The model under review builds one solid part; all positions refer to its coordinate system, in mm. Face numbers are marked on the shaded views. Give positions to 0.01 mm unless a question says otherwise; leave off trailing zeros. Write each loop counter-clockwise with the first axis right and the second up, starting at its lowest first coordinate (ties: lowest second). Pieces come first, ordered by that corner, then holes. Notation, with made-up numbers: (9, 79.25) -> (16, 79.25) arc R23 cw to (16, 106.25) -> close; hole circle Ø10 at (-0.75, 6). An arc over 180 degrees is marked (long way). Use CSV: the item, a comma, the result in double quotes.
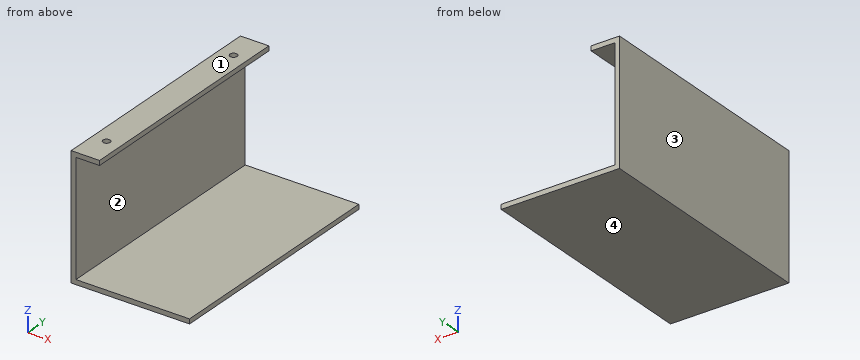
```python
from build123d import *

# Parameters (mm, degrees)
F0_W     = 50
F0_H     = 100
F1_DEPTH = 2
F2_W     = 2
F2_H     = 100
F3_DEPTH = 50
F4_W     = 100
F4_H     = 2
F5_DEPTH = 10
F6_R     = 1.5
F7_DEPTH = 2


with BuildPart() as f1:
    # F0 (on Top) → F1 (new body)
    with BuildSketch(Plane.XY):
        Rectangle(F0_W, F0_H)
    extrude(amount=F1_DEPTH)

    # F2 (on face) → F3 (join)
    with BuildSketch(Plane.XY.offset(2)):
        with Locations((-24, 0)):
            Rectangle(F2_W, F2_H)
    extrude(amount=F3_DEPTH)

    # F4 (on face) → F5 (join)
    with BuildSketch(Plane.YZ.offset(-23)):
        with Locations((0, 51)):
            Rectangle(F4_W, F4_H)
    extrude(amount=F5_DEPTH)

    # F6 (on face) → F7 (cut, through all)
    with BuildSketch(Plane.XY.offset(52)):
        with Locations((-18.9944, 37.5)):
            Circle(F6_R)
        with Locations((-18.9944, -37.5)):
            Circle(F6_R)
    extrude(amount=-F7_DEPTH, mode=Mode.SUBTRACT)


solid = f1.part
```
Q1. Consider section B-B (y = 25.5). Write out the cut boundary in (x, z), then the cut area to 3 significant figures.
Derived:
outline,"(-25, 0) -> (25, 0) -> (25, 2) -> (-23, 2) -> (-23, 50) -> (-13, 50) -> (-13, 52) -> (-25, 52) -> close"
area,"220 mm2"
Q2. The part is to be moulded in two halves that separate along Z. For the marked faces 1, 2, 3 and 4, say which applies: pulls with the +Z half, pulls with the -Z half, needs draft (parallel to the pull), parting line crosses it, or undercut.
Derived:
face 1,"pulls with the +Z half"
face 2,"undercut"
face 3,"needs draft"
face 4,"pulls with the -Z half"
Q3. Consider section C-C (x = -19). Write out the cut boundary in (y, z).
Derived:
outline,"(-50, 0) -> (50, 0) -> (50, 2) -> (-50, 2) -> close; (-50, 50) -> (-39, 50) -> (-39, 52) -> (-50, 52) -> close; (-36, 50) -> (36, 50) -> (36, 52) -> (-36, 52) -> close; (39, 50) -> (50, 50) -> (50, 52) -> (39, 52) -> close"
Q4. To check wall thickness, follow probe 1 along X at (y, z) = (1, 34); probe 2 along Z at (x, y) = (19, 27.5). State the ranges of each line that lie inside material, in increasing order.
Derived:
probe 1,"x = -25 to -23"
probe 2,"z = 0 to 2"
Q5. Consider section A-A (y = 37.5). Write out the cut boundary in (x, z), then the cut area to 3 significant figures.
Derived:
outline,"(-25, 0) -> (25, 0) -> (25, 2) -> (-23, 2) -> (-23, 50) -> (-20.49, 50) -> (-20.49, 52) -> (-25, 52) -> close; (-17.49, 50) -> (-13, 50) -> (-13, 52) -> (-17.49, 52) -> close"
area,"214 mm2"
Q6. Consider section D-D (z = 10). Write out the cut boundary in (x, y), then the cut area to 3 significant figures.
Derived:
outline,"(-25, -50) -> (-23, -50) -> (-23, 50) -> (-25, 50) -> close"
area,"200 mm2"
Q7. Insertion check: pin 1 (5 mm diameter, centred on x = 9, y = -5, fed in from -Z); pin 2 (4 mm diameter, centred on y = -10.5, z = 13, fed in from +X); pin 3 (6 mm diameter, centred on x = 0.5, y = -13, fed in from +Z); pin 4 (2 mm diameter, centred on y = -22.5, z = 51.5, fed in from +X). Each pin has a flat end and moves straight along its axis. Give the tip position at first contact, or say it passes through.
Derived:
pin 1,"stops at z = 0"
pin 2,"stops at x = -23"
pin 3,"stops at z = 2"
pin 4,"stops at x = -13"
